Could you check a few things on this model? Use its own coordinates, in mm. Coordinates: 2 decimals unless noted, no trailing zeros. Loops run counter-clockwise (first coordinate to the right, second up) from the corner with the lowest first, then second, coordinate; pieces in that order, holes last. Notation, with made-up numbers: M -32,58 L -14,58 A29 cw -14,78 Z; hole C 37.25,-29 d7. An arc over 180 degrees is marked long. Return JSON: item names as keys, results as strings. Group by question number.
Autodesk Inventor part; units mm, degrees
ref_plane "YZ Plane" through (0, 0, 0) normal (1, 0, 0) x (0, 1, 0)
ref_plane "XZ Plane" through (0, 0, 0) normal (0, 1, 0) x (-1, 0, 0)
ref_plane "XY Plane" through (0, 0, 0) normal (0, 0, 1) x (1, 0, 0)
sketch "Sketch1" plane through (0, 0, 0) normal (0, 0, 1) x (1, 0, 0)
  arc A0 (-16.0194, 6.752) -> (-16.0208, -6.1468) centre (-16.0175, 0.3026) ccw
  arc A1 (649.005, -6.4829) -> (649.0007, 6.9464) centre (649.0026, 0.2317) ccw
  line L0 (649.005, -6.4829) -> (-16.0208, -6.1468)
  arc A2 (649.0045, -7.4829) -> (649.0008, 7.9464) centre (649.0026, 0.2317) ccw
  line L1 (649.0008, 7.9464) -> (311.9827, 7.8478)
  line L2 (649.0045, -7.4829) -> (-16.0213, -7.1468)
  arc A3 (-16.0124, 7.7519) -> (-16.0213, -7.1468) centre (-16.0175, 0.3026) ccw
  line L3 (312.9758, 5.1048) -> (312.9758, 3.1737)
  line L4 (312.9758, 3.1737) -> (313.0166, 2.6809)
  line L5 (313.0166, 2.6809) -> (313.1377, 2.2016)
  line L6 (313.1377, 2.2016) -> (313.3359, 1.7486)
  line L7 (313.3359, 1.7486) -> (313.6059, 1.3343)
  line L8 (313.6059, 1.3343) -> (313.9402, 0.97)
  line L9 (313.9402, 0.97) -> (314.3298, 0.6656)
  line L10 (314.3298, 0.6656) -> (314.7641, 0.4293)
  line L11 (314.7641, 0.4293) -> (315.2314, 0.2675)
  line L12 (315.2314, 0.2675) -> (315.7189, 0.1847)
  line L13 (315.7189, 0.1847) -> (316.2133, 0.1831)
  line L14 (316.2133, 0.1831) -> (318.2319, 0.3939)
  line L15 (318.2319, 0.3939) -> (320.8327, 0.8165)
  line L16 (320.8327, 0.8165) -> (323.4008, 1.4058)
  line L17 (323.4008, 1.4058) -> (325.9257, 2.1591)
  line L18 (325.9257, 2.1591) -> (326.3565, 2.3413)
  line L19 (326.3565, 2.3413) -> (326.7537, 2.5883)
  line L20 (326.7537, 2.5883) -> (327.1077, 2.8941)
  line L21 (327.1077, 2.8941) -> (327.4099, 3.2511)
  line L22 (327.4099, 3.2511) -> (327.6529, 3.6508)
  line L23 (327.6529, 3.6508) -> (327.8308, 4.0834)
  line L24 (327.8308, 4.0834) -> (327.9394, 4.5384)
  line L25 (327.9394, 4.5384) -> (327.9758, 5.0047)
  line L26 (327.9758, 5.1048) -> (327.9758, 5.0047)
  line L27 (312.9758, 5.1048) -> (327.9758, 5.1048)
  line L28 (308.2722, 6.8467) -> (308.2722, 3.2511)
  line L29 (308.2722, 3.2511) -> (307.9758, 1.1103)
  line L30 (307.9758, 1.1103) -> (306.659, 0.0522)
  line L31 (306.659, 0.0522) -> (304.4805, -0.3835)
  line L32 (304.4805, -0.3835) -> (297.6339, 0.7991)
  line L33 (297.6339, 0.7991) -> (293.4637, 2.2307)
  line L34 (293.4637, 2.2307) -> (291.5964, 4.3469)
  line L35 (291.5964, 4.3469) -> (289.9159, 5.7785)
  line L36 (289.9159, 5.7785) -> (288.4843, 6.3387)
  line L37 (288.4843, 6.3387) -> (285.1855, 6.4631)
  line L38 (285.1855, 6.4631) -> (276.9073, 6.3387)
  line L39 (276.9073, 6.3387) -> (272.4922, 5.7434)
  line L40 (272.4922, 5.7434) -> (272.7903, 5.0479)
  line L41 (272.7903, 5.0479) -> (277.3612, 5.5944)
  line L42 (277.3612, 5.5944) -> (285.9563, 5.7931)
  line L43 (285.9563, 5.7931) -> (288.9373, 5.5944)
  line L44 (288.9373, 5.5944) -> (290.6266, 4.4517)
  line L45 (290.6266, 4.4517) -> (291.4215, 3.1599)
  line L46 (291.4215, 3.1599) -> (293.4088, 1.3216)
  line L47 (293.4088, 1.3216) -> (297.5325, 0.0795)
  line L48 (297.5325, 0.0795) -> (302.7492, -0.9638)
  line L49 (302.7492, -0.9638) -> (305.929, -1.0135)
  line L50 (305.929, -1.0135) -> (308.7609, 0.1789)
  line L51 (308.7609, 0.1789) -> (309.4068, 2.0172)
  line L52 (309.4068, 2.0172) -> (309.3584, 4.7043)
  line L53 (309.3584, 4.7043) -> (309.1601, 6.2436)
  line L54 (309.1601, 6.2436) -> (308.9658, 7.7519)
  line L55 (312.672, 6.848) -> (312.672, 3.2511)
  line L56 (312.672, 3.2511) -> (312.9684, 1.1103)
  line L57 (312.9684, 1.1103) -> (314.2852, 0.0522)
  line L58 (314.2852, 0.0522) -> (316.4637, -0.3835)
  line L59 (316.4637, -0.3835) -> (323.3103, 0.7991)
  line L60 (323.3103, 0.7991) -> (327.4805, 2.2307)
  line L61 (327.4805, 2.2307) -> (329.3478, 4.3469)
  line L62 (329.3478, 4.3469) -> (331.0283, 5.7785)
  line L63 (331.0283, 5.7785) -> (332.4599, 6.3387)
  line L64 (332.4599, 6.3387) -> (335.7587, 6.4631)
  line L65 (335.7587, 6.4631) -> (344.0369, 6.3387)
  line L66 (344.0369, 6.3387) -> (348.452, 5.7434)
  line L67 (348.452, 5.7434) -> (348.156, 5.0487)
  line L68 (348.156, 5.0487) -> (343.5851, 5.5953)
  line L69 (343.5851, 5.5953) -> (334.9899, 5.794)
  line L70 (334.9899, 5.794) -> (332.009, 5.5953)
  line L71 (332.009, 5.5953) -> (330.3197, 4.4525)
  line L72 (330.3197, 4.4525) -> (329.5248, 3.1608)
  line L73 (329.5248, 3.1608) -> (327.5375, 1.3225)
  line L74 (327.5375, 1.3225) -> (323.4138, 0.0804)
  line L75 (323.4138, 0.0804) -> (318.197, -0.9629)
  line L76 (318.197, -0.9629) -> (315.0173, -1.0126)
  line L77 (315.0173, -1.0126) -> (312.1854, 0.1798)
  line L78 (312.1854, 0.1798) -> (311.5395, 2.0181)
  line L79 (311.5395, 2.0181) -> (311.5892, 4.8003)
  line L80 (311.5892, 4.8003) -> (311.7879, 6.3395)
  line L81 (311.5892, 4.8003) -> (311.9827, 7.8478)
  line L82 (-16.0194, 6.752) -> (308.2722, 6.8467)
  line L83 (312.672, 6.848) -> (649.0007, 6.9464)
  line L84 (308.9658, 7.7519) -> (-16.0124, 7.7519)
  point P0 (0, 0)
  dimension "d1" = 1
extrude "Extrusion1" add sketch "Sketch1" along normal blind 5 contours A0 L0 A1 L83 L55 L56 L57 L58 L59 L60 L61 L62 L63 L64 L65 L66 L67 L68 L69 L70 L71 L72 L73 L74 L75 L76 L77 L78 L79 L80 L81 L1 A2 L2 A3 L84 L54 L53 L52 L51 L50 L49 L48 L47 L46 L45 L44 L43 L42 L41 L40 L39 L38 L37 L36 L35 L34 L33 L32 L31 L30 L29 L28 L82
properties part number "YBELT"
(1) Will these pins go through, and if not, where does the flat tip stop? P1, Ø1.1, axis at y = 5, z = 2, coming from the -X side; P2, Ø2.5, axis at x = 476, z = 2.5, coming from the +Y side; P3, Ø1.5, axis at y = -6, z = 3.5, coming from the -X side.
(2) Imagine slicing it at A-A, the plane y = -3.75. Write out the boundary of the cut face in (x, z), then the cut area to 3 significant figures.
(3) If I drill on L1, parallel to Y at x = 34, z = 1; L2, parallel to Y at x = 483, z = 3.8; L3, parallel to X at y = 2.5, z = 1.65, over which ranges is the centre line in solid material (lowest first)? Write a range as [from, to].
(4) Imagine slicing it at B-B, the plane x = 207.5. Write out the boundary of the cut face in (y, z), then the cut area to 3 significant figures.
Checks:
{
 "1": {"P1": "x = -22.21", "P2": "y = 7.9", "P3": "x = -20.98"},
 "2": {"outline": "M -22.27,0 L -21.03,0 L -21.03,5 L -22.27,5 Z; M 654.41,0 L 655.61,0 L 655.61,5 L 654.41,5 Z", "area": "12.2 mm²"},
 "3": {"L1": "[-7.17, -6.17], [6.77, 7.75]", "L2": "[-7.4, -6.4], [6.9, 7.9]", "L3": "[-23.14, -22.08], [292.13, 293.23], [308.17, 309.4], [311.55, 312.78], [327.72, 328.81], [655.32, 656.38]"},
 "4": {"outline": "M -7.26,0 L -6.26,0 L -6.26,5 L -7.26,5 Z; M 6.82,0 L 7.75,0 L 7.75,5 L 6.82,5 Z", "area": "9.67 mm²"}
}
